Input: part model. Units: mm. Frame: model coordinates. A direction names the side the tool comes from. Coordinates: 2 decimals unless noted, no trailing zeros. Loops run counter-clockwise (first coordinate to the right, second up) from the corner with the lowest first, then second, coordinate; pieces in that order, holes last.
(1) Set-up query: faces 4 (the face through (1.4, -1.4, 6)), 5 (the face through (0.74, -1.305, 4.986)), 6 (the face through (2, 0, -2)). Return all of +Z, -Z, +X, -X, +Y, -Y with unobstructed straight access to the full face (end or side cutting, diameter ignored); none if empty.
(2) Line query: L1, parallel to Z at x = 1.25, y = -3; L2, parallel to X at y = 0.5, z = 5; L3, parallel to X at y = 1.25, z = 4.25. Output: solid intervals per line, ascending.
(3) Section A-A, the plane y = 0. Return loops of the section in (x, z), then the cut area to 3 significant figures.
(4) Contact query for flat-ended pins moving along their axis: P1, Ø1, axis at x = -0.5, y = 0, coming from the +Z side; P2, Ø1.5, axis at y = 1, z = 1, coming from the -X side. Output: stop coordinate, or through.
(5) Section B-B, the plane z = 4.5. Return loops of the section in (x, y), then the cut area to 3 significant figures.
(6) Mould query, pull axis X, two halves, no side actions, for faces 1 (the face through (0, 0, -6)), 2 (the face through (0, 0, 4)), 3 (the face through (1.341, 3.233, 3.975)). Classes: released by +X, released by -X, zero draft, split by the parting line, or undercut.
(7) Section C-C, the plane z = -0.5. Return loops of the section in (x, y).
```python
from build123d import *

# Parameters (mm, degrees)
CUT_EXTRUDE1_START = -2
CUT_EXTRUDE1_DEPTH = 2
SKETCH4_R          = 1.732050808
CUT_EXTRUDE2_DEPTH = 0.5
CUT_EXTRUDE2_TAPER = 45


with BuildPart() as part:
    # Sketch2 → Revolve1 (revolve)
    with BuildSketch(Plane(origin=(0, 0, 0), x_dir=(0, 0, -1), z_dir=(1, 0, 0))):
        Polygon((-5.8, 3.5), (-2.2, 3.5), (-2, 3.3), (-2, 2), (5.3, 2), (6, 1.3), (6, 0), (-6, 0), (-6, 3.3), align=None)
    revolve(axis=Axis((0, 0, -6), (0, 0, 1)))

    # Sketch3 → Cut-Extrude1 (cut)
    with BuildSketch(Plane.XY.offset(6).offset(CUT_EXTRUDE1_START)):
        Polygon((0, 1.732050808), (-1.5, 0.866025404), (-1.5, -0.866025404), (0, -1.732050808), (1.5, -0.866025404), (1.5, 0.866025404), align=None)
    extrude(amount=CUT_EXTRUDE1_DEPTH, mode=Mode.SUBTRACT)

    # Sketch4 → Cut-Extrude2 (cut)
    with BuildSketch(Plane.XY.offset(6)):
        Circle(SKETCH4_R)
    extrude(amount=-CUT_EXTRUDE2_DEPTH, taper=CUT_EXTRUDE2_TAPER, mode=Mode.SUBTRACT)


solid = part.part
```
Report:
1. face 4: +Z, +X, -X, +Y, -Y
1. face 5: +Z
1. face 6: -Z
2. L1: z = 2 to 6
2. L2: x = -3.46 to -1.5, 1.5 to 3.46
2. L3: x = -3.27 to -0.83, 0.83 to 3.27
3. outline: (-3.5, 2.2) - (-3.3, 2) - (-2, 2) - (-2, -5.3) - (-1.3, -6) - (1.3, -6) - (2, -5.3) - (2, 2) - (3.3, 2) - (3.5, 2.2) - (3.5, 5.8) - (3.3, 6) - (1.73, 6) - (1.5, 5.77) - (1.5, 4) - (-1.5, 4) - (-1.5, 5.77) - (-1.73, 6) - (-3.3, 6) - (-3.5, 5.8) - close
3. area: 53.4 mm2
4. P1: stops at z = 4
4. P2: stops at x = -1.98
5. outline: circle Ø7 at (0, 0); hole (-1.5, -0.87) - (0, -1.73) - (1.5, -0.87) - (1.5, 0.87) - (0, 1.73) - (-1.5, 0.87) - close
5. area: 30.7 mm2
6. face 1: zero draft
6. face 2: undercut
6. face 3: split by the parting line
7. outline: circle Ø4 at (0, 0)
